```python
from build123d import *

# Parameters (mm, degrees)
SKETCH1_R           = 76
BOSS_EXTRUDE1_DEPTH = 18
CUT_EXTRUDE4_DEPTH  = 8.89
SKETCH5_R           = 3
CUT_EXTRUDE5_DEPTH  = 20
CUT_EXTRUDE6_DEPTH  = 10.11
CUT_EXTRUDE7_DEPTH  = 10.11


with BuildPart() as part:
    # Sketch1 → Boss-Extrude1 (new body)
    with BuildSketch(Plane(origin=(0, 0, 0), x_dir=(1, 0, 0), z_dir=(0, 1, 0))):
        Circle(SKETCH1_R)
    extrude(amount=BOSS_EXTRUDE1_DEPTH)

    # Sketch2 → Cut-Extrude4 (cut)
    with BuildSketch(Plane(origin=(0, 18, 0), x_dir=(1, 0, 0), z_dir=(0, 1, 0))):
        with BuildLine():
            Line((-58.007955522, 49.931796385), (58.007955522, 49.931796385))
            ThreePointArc((58.007955522, 49.931796385), (107.939751907, 0), (58.007955522, -49.931796385))
            Line((58.007955522, -49.931796385), (-58.007955522, -49.931796385))
            ThreePointArc((-58.007955522, -49.931796385), (-107.939751907, 0), (-58.007955522, 49.931796385))
        make_face()
    extrude(amount=-CUT_EXTRUDE4_DEPTH, mode=Mode.SUBTRACT)

    # Sketch5 → Cut-Extrude5 (cut)
    with BuildSketch(Plane(origin=(0, 9.11, 0), x_dir=(1, 0, 0), z_dir=(0, 1, 0))):
        Circle(SKETCH5_R)
    extrude(amount=-CUT_EXTRUDE5_DEPTH, mode=Mode.SUBTRACT)

    # Sketch7 → Cut-Extrude6 (cut, through all)
    with BuildSketch(Plane(origin=(0, 9.11, 0), x_dir=(1, 0, 0), z_dir=(0, 1, 0))):
        Polygon((-50.125135648, 42.322849323), (-67.902913426, 6.490592664), (-22.902913426, 6.490592664), align=None)
        Polygon((67.902913426, 6.490592664), (22.902913426, 6.490592664), (50.125135648, 42.322849323), align=None)
        Polygon((50.125135648, -42.322849323), (67.902913426, -6.490592664), (22.902913426, -6.490592664), align=None)
        Polygon((-67.902913426, -6.490592664), (-22.902913426, -6.490592664), (-50.125135648, -42.322849323), align=None)
    extrude(amount=-CUT_EXTRUDE6_DEPTH, mode=Mode.SUBTRACT)

    # Sketch9 → Cut-Extrude7 (cut, through all)
    with BuildSketch(Plane(origin=(0, 9.11, 0), x_dir=(1, 0, 0), z_dir=(0, 1, 0))):
        Polygon((-12.5, 6.490592664), (-12.5, 42.322849323), (-39.5, 42.322849323), align=None)
        Polygon((12.5, 6.490592664), (39.5, 42.322849323), (12.5, 42.322849323), align=None)
        Polygon((12.5, -6.490592664), (12.5, -42.322849323), (39.5, -42.322849323), align=None)
        Polygon((-12.5, -6.490592664), (-39.5, -42.322849323), (-12.5, -42.322849323), align=None)
    extrude(amount=-CUT_EXTRUDE7_DEPTH, mode=Mode.SUBTRACT)


solid = part.part
```
CAD build for the part. Positions are in the model's coordinates, mm. A direction names the side the tool comes from. Give positions to 0.01 mm unless a question says otherwise; leave off trailing zeros. Loops run counter-clockwise (first coordinate to the right, second up) from the corner with the lowest first, then second, coordinate; pieces in that order, holes last. Notation, with made-up numbers: (19, 83) -> (59, 83) arc R15 cw to (59, 101) -> close; hole circle Ø1 at (0.5, -3). An arc over 180 degrees is marked (long way). Use a Markdown table: item, result.
1. Flat gauge pins, fed straight in: pin 1 (2.5 mm diameter, centred on x = -53, y = 5.5, fed in from -Z); pin 2 (4.5 mm diameter, centred on x = 52, y = 6.5, fed in from +Z); pin 3 (4.5 mm diameter, centred on y = 6, z = 28.5, fed in from -X). Where does each tip first touch, or does it go through?
Check result:
| item | result |
|---|---|
| pin 1 | stops at z = -55.66 |
| pin 2 | stops at z = 57.45 |
| pin 3 | stops at x = -71.32 |
2. Which spindle directions (+Z, -Z, +X, -X, +Y, -Y) get a long thin tool onto all of the face, cutting with end or side? Do faces 3 (the flat face through (-1, 18, -60)), 4 (the flat face through (12.5, 5, 24)), 5 (the flat face through (1, 14, 49.932)). Say none if no direction does.
Check result:
| item | result |
|---|---|
| face 3 | +Z, -Z, +X, -X, +Y |
| face 4 | +Y, -Y |
| face 5 | +X, -X, +Y |
3. Slice it at B-B (z = 0). List the corners of the cut face in (x, y), plus the area to 3 significant figures.
Check result:
| item | result |
|---|---|
| outline | (-76, 0) -> (-3, 0) -> (-3, 9.11) -> (-76, 9.11) -> close; (3, 0) -> (76, 0) -> (76, 9.11) -> (3, 9.11) -> close |
| area | 1,330 mm^2 |
4. Slice it at C-C (x = 43.5). List the corners of the cut face in (y, z), plus the area to 3 significant figures.
Check result:
| item | result |
|---|---|
| outline | (0, -62.32) -> (18, -62.32) -> (18, -49.93) -> (9.11, -49.93) -> (9.11, -33.6) -> (0, -33.6) -> close; (0, -6.49) -> (9.11, -6.49) -> (9.11, 6.49) -> (0, 6.49) -> close; (0, 33.6) -> (9.11, 33.6) -> (9.11, 49.93) -> (18, 49.93) -> (18, 62.32) -> (0, 62.32) -> close |
| area | 862 mm^2 |
5. Mould opens along X. For faces 1 (the flat face through (-12.5, 5, 25)), 2 (the flat face through (1, 9.11, 10)) say: pulls with the +X half, pulls with the -X half, needs draft (parallel to the pull), parting line crosses it, or undercut.
Check result:
| item | result |
|---|---|
| face 1 | undercut |
| face 2 | needs draft |
6. Wall check: L1, parallel to Z at x = 0, y = 3.75; L2, parallel to X at y = 7.75, z = -16. Give the ranges that are in metal, low to high. Write a range as [from, to].
Check result:
| item | result |
|---|---|
| L1 | z = [-76, -3], [3, 76] |
| L2 | x = [-74.3, -63.18], [-30.13, -19.67], [-12.5, 12.5], [19.67, 30.13], [63.18, 74.3] |
7. Slice it at D-D (z = -30.5). List the corners of the cut face in (x, y), plus the area to 3 significant figures.
Check result:
| item | result |
|---|---|
| outline | (-69.61, 0) -> (-55.99, 0) -> (-55.99, 9.11) -> (-69.61, 9.11) -> close; (-41.14, 0) -> (-30.59, 0) -> (-30.59, 9.11) -> (-41.14, 9.11) -> close; (-12.5, 0) -> (12.5, 0) -> (12.5, 9.11) -> (-12.5, 9.11) -> close; (30.59, 0) -> (41.14, 0) -> (41.14, 9.11) -> (30.59, 9.11) -> close; (55.99, 0) -> (69.61, 0) -> (69.61, 9.11) -> (55.99, 9.11) -> close |
| area | 668 mm^2 |
8. Slice it at A-A (x = 0). List the corners of the cut face in (y, z).
Check result:
| item | result |
|---|---|
| outline | (0, -76) -> (18, -76) -> (18, -49.93) -> (9.11, -49.93) -> (9.11, -3) -> (0, -3) -> close; (0, 3) -> (9.11, 3) -> (9.11, 49.93) -> (18, 49.93) -> (18, 76) -> (0, 76) -> close |
